from build123d import *

# Parameters (mm, degrees)
F1_DEPTH = 7
F2_R     = 5.08


with BuildPart() as f1:
    # F0 (on Top) → F1 (new body)
    with BuildSketch(Plane.XY):
        with BuildLine():
            Line((-14.855128, 8.576612), (-29.004115, 1.684053))
            ThreePointArc((-29.004115, 1.684053), (-35.87974, -20.654294), (-13.131215, -26.019049))
            Line((-13.131215, -26.019049), (0, -17.27825))
            Line((0, -17.27825), (13.131215, -26.019049))
            ThreePointArc((13.131215, -26.019049), (35.640928, -21.0573), (29.833927, 1.249311))
            Line((29.833927, 1.249311), (16.048566, 8.994085))
            Line((16.048566, 8.994085), (15.99993, 25.447296))
            ThreePointArc((15.99993, 25.447296), (-0.585843, 41.389271), (-15.96049, 24.276274))
            Line((-15.96049, 24.276274), (-14.855128, 8.576612))
        make_face()
        with BuildLine():
            ThreePointArc((-11.202065, -12.7), (-32.424195, -15.493946), (-12.648318, -7.30251))
            ThreePointArc((-12.648318, -7.30251), (-11.569895, -9.906054), (-11.202065, -12.7))
        make_face(mode=Mode.SUBTRACT)
        with BuildLine():
            ThreePointArc((32.997045, -12.7), (19.150036, -23.325184), (12.470766, -7.2))
            ThreePointArc((12.470766, -7.2), (24.844055, -2.074816), (32.997045, -12.7))
        make_face(mode=Mode.SUBTRACT)
        with BuildLine():
            ThreePointArc((-9.526279, -5.5), (-9.526279, 5.5), (0, 11))
            ThreePointArc((0, 11), (7.778175, 7.778175), (11, 0))
            ThreePointArc((11, 0), (10.625184, -2.847009), (9.526279, -5.5))
            ThreePointArc((9.526279, -5.5), (0, -11), (-9.526279, -5.5))
        make_face(mode=Mode.SUBTRACT)
        with BuildLine():
            ThreePointArc((0, 14.4), (-7.778175, 33.178175), (11, 25.4))
            ThreePointArc((11, 25.4), (7.778175, 17.621825), (0, 14.4))
        make_face(mode=Mode.SUBTRACT)
    extrude(amount=F1_DEPTH)

    # F2
    f2_edges = [f1.edges().sort_by_distance(p)[0] for p in [
        (-14.855128, 8.576612, 3.5),
        (16.048566, 8.994085, 3.5),
        (0, -17.27825, 3.5),
    ]]
    fillet(f2_edges, radius=F2_R)


solid = f1.part
Here's how the part is built. I have some questions about the finished solid (model axes, mm). A direction names the side the tool comes from. Give positions to 0.01 mm unless a question says otherwise; leave off trailing zeros. Write each loop counter-clockwise with the first axis right and the second up, starting at its lowest first coordinate (ties: lowest second). Pieces come first, ordered by that corner, then holes. Notation, with made-up numbers: (-23, 21.5) -> (6, 21.5) arc R24 ccw to (6, 35.5) -> close; hole circle Ø8 at (-6, 22.5). An arc over 180 degrees is marked (long way). Use one line per item in the form item = value. Start each with the question number.
1. If I drill on L1, parallel to X at y = -12.7, z = 1.5; L2, parallel to Y at x = 4, z = 1.5; L3, parallel to Y at x = -3.5, z = 4.5, over which ranges is the centre line in solid material (lowest first)?
2. Imagine slicing it at D-D on y = -22. List the corners of the cut face in (x, z) for me, plus the area to 3 significant figures.
3. Imagine slicing it at C-C on z = 5. List the corners of the cut face in (x, y) for me.
4. Will these pins go through, and if not, where does the flat tip stop? pin 1 Ø4 at (y, z) = (1.5, 3) entering from -X; pin 2 Ø1 at (y, z) = (-13.5, 5.5) entering from +X; pin 3 Ø13 at (x, y) = (0, 25.4) entering from -Z; pin 4 Ø3 at (y, z) = (24, 5.5) entering from +X.
5. Imagine slicing it at A-A on x = 7. List the corners of the cut face in (y, z) for me, plus the area to 3 significant figures.
6. Imagine slicing it at B-B on y = 28.5. List the corners of the cut face in (x, z) for me, plus the area to 3 significant figures.
7. On a 3-axis mill with a long thin cutter (end or side, diameter ignored), from which of +Z, -Z, +X, -X, +Y, -Y can I reach the whole of each face in a straight line? I mean faces 1 (the face through (7.901, -22.537, 3.451)), 2 (the face through (-23.39, 4.42, 3.45)), 3 (the face through (-15.79, 9.06, 3.55)). Say none if no direction works.
Entries:
q1.L1 = -38 to -32.79, -11.2 to 11, 33 to 38
q1.L2 = -19.94 to -10.25, 10.25 to 15.15, 35.65 to 40.89
q1.L3 = -19.61 to -10.43, 10.43 to 14.97, 35.83 to 41.01
q2.outline = (-35.02, 0) -> (-27.48, 0) -> (-27.48, 7) -> (-35.02, 7) -> close; (-16.52, 0) -> (-7.09, 0) -> (-7.09, 7) -> (-16.52, 7) -> close; (7.09, 0) -> (16.12, 0) -> (16.12, 7) -> (7.09, 7) -> close; (27.87, 0) -> (35.02, 0) -> (35.02, 7) -> (27.87, 7) -> close
q2.area = 232 mm²
q3.outline = (-29, 1.68) arc R16 ccw (long way) to (-13.13, -26.02) -> (-2.81, -19.15) arc R5.08 cw to (2.81, -19.15) -> (13.13, -26.02) arc R16 ccw (long way) to (29.83, 1.25) -> (18.63, 7.54) arc R5.08 cw to (16.04, 11.96) -> (16, 25.45) arc R16 ccw (long way) to (-15.96, 24.28) -> (-15.1, 12) arc R5.08 cw to (-17.94, 7.07) -> close; hole (-12.65, -7.3) arc R10.79 ccw (long way) to (-11.2, -12.7) arc R10.79 ccw to start; hole (0, 11) arc R11 ccw (long way) to (9.53, -5.5) arc R11 ccw to (11, 0) arc R11 ccw to start; hole (0, 14.4) arc R11 ccw to (11, 25.4) arc R11 ccw (long way) to start; hole circle Ø22 at (22, -12.7)
q4.pin_1 = -32.35
q4.pin_2 = 37.99
q4.pin_3 = through
q4.pin_4 = 16.01
q5.outline = (-21.94, 0) -> (-8.49, 0) -> (-8.49, 7) -> (-21.94, 7) -> close; (8.49, 0) -> (16.91, 0) -> (16.91, 7) -> (8.49, 7) -> close; (33.89, 0) -> (39.79, 0) -> (39.79, 7) -> (33.89, 7) -> close
q5.area = 194 mm²
q6.outline = (-15.7, 0) -> (-10.55, 0) -> (-10.55, 7) -> (-15.7, 7) -> close; (10.55, 0) -> (15.7, 0) -> (15.7, 7) -> (10.55, 7) -> close
q6.area = 72.0 mm²
q7.face_1 = +Z, -Z, -Y
q7.face_2 = +Z, -Z, -X, +Y
q7.face_3 = +Z, -Z, -X
